Part model, mm, in its own coordinate system. Give positions to 0.01 mm unless a question says otherwise; leave off trailing zeros. Write each loop counter-clockwise with the first axis right and the second up, starting at its lowest first coordinate (ties: lowest second). Pieces come first, ordered by that corner, then holes.
Autodesk Inventor part; units mm, degrees
ref_plane "YZ Plane" through (0, 0, 0) normal (1, 0, 0) x (0, 1, 0)
ref_plane "XZ Plane" through (0, 0, 0) normal (0, 1, 0) x (-1, 0, 0)
ref_plane "XY Plane" through (0, 0, 0) normal (0, 0, 1) x (1, 0, 0)
sketch "Sketch1" plane through (0, 0, 0) normal (0, 1, 0) x (-1, 0, 0)
  line L0 (4.1559, 203.2) -> (4.1559, -203.2)
  line L1 (4.1559, -203.2) -> (156.5559, -291.1882)
  line L2 (4.1559, 203.2) -> (156.5559, 291.1882)
  line L3 (4.1559, 203.2) -> (180.1322, 203.2) construction
  line L4 (156.5559, 291.1882) -> (156.5559, -291.1882)
  point P0 (0, 0)
  point P1 (4.1559, 0)
  dimension "d0" = 120
  dimension "d1" = 30
  dimension "d2" = 406.4
  dimension "d5" = 152.4
extrude "Extrusion1" add sketch "Sketch1" along normal blind 6.35
sketch "Sketch4" plane through (0, 6.35, 0) normal (0, 1, 0) x (1, 0, 0)
  line L0 (-4.1559, -203.2) -> (-4.1559, 203.2)
  point P0 (0, 0)
  point P1 (-80.3559, 0)
  dimension "d12" = 76.2
  dimension "d13" = 203.2
hole "Hole1" at (-80.3559, 6.35, 0) direction (0, -1, 0) diameter 13.4925 end through all
sketch "Sketch5" plane through (0, 6.35, 0) normal (0, 1, 0) x (1, 0, 0)
  line L0 (-1271.2154, -905.4078) -> (-39.3808, -194.2078)
  line L1 (-1258.5154, -927.4048) -> (-1271.2154, -905.4078)
  line L2 (-1258.5154, -927.4048) -> (-26.6808, -216.2048)
  line L3 (-39.3808, -194.2078) -> (-26.6808, -216.2048)
  circle A0 centre (-1049.6741, -711.3284) radius 3.3782
  circle A1 centre (-248.9471, -249.0284) radius 3.3782
  circle A2 centre (-318.2291, -289.0284) radius 3.3782
  circle A3 centre (-1118.9562, -751.3284) radius 3.3782
  line L4 (-127.679, -193.6709) -> (-1227.5312, -828.6709)
  line L5 (-140.379, -171.6739) -> (-127.679, -193.6709)
  line L6 (-140.379, -171.6739) -> (-1240.2312, -806.6739)
  line L7 (-1227.5312, -828.6709) -> (-1240.2312, -806.6739)
  circle A4 centre (-318.2291, 289.0284) radius 3.3782
  circle A5 centre (-1118.9562, 751.3284) radius 3.3782
  circle A6 centre (-1049.6741, 711.3284) radius 3.3782
  circle A7 centre (-248.9471, 249.0284) radius 3.3782
  line L8 (-1227.5312, 828.6709) -> (-127.679, 193.6709)
  line L9 (-1240.2312, 806.6739) -> (-1227.5312, 828.6709)
  line L10 (-1240.2312, 806.6739) -> (-140.379, 171.6739)
  line L11 (-127.679, 193.6709) -> (-140.379, 171.6739)
  line L12 (-39.3808, 194.2078) -> (-1271.2154, 905.4078)
  line L13 (-26.6808, 216.2048) -> (-39.3808, 194.2078)
  line L14 (-26.6808, 216.2048) -> (-1258.5154, 927.4048)
  line L15 (-1271.2154, 905.4078) -> (-1258.5154, 927.4048)
  line L16 (-156.5559, -291.1882) -> (-26.6808, -216.2048)
  line L17 (-39.3808, -194.2078) -> (-156.5559, -261.8588)
  line L18 (-156.5559, 291.1882) -> (-156.5559, -291.1882)
  line L19 (-156.5559, -261.8588) -> (-156.5559, -291.1882)
  line L20 (-156.5559, -210.343) -> (-127.679, -193.6709)
  line L21 (-127.679, -193.6709) -> (-140.379, -171.6739)
  line L22 (-140.379, -171.6739) -> (-156.5559, -181.0136)
  line L23 (-156.5559, -181.0136) -> (-156.5559, -210.343)
  line L24 (-39.3808, -194.2078) -> (-26.6808, -216.2048)
  line L25 (-156.5559, 181.0136) -> (-140.379, 171.6739)
  line L26 (-140.379, 171.6739) -> (-127.679, 193.6709)
  line L27 (-127.679, 193.6709) -> (-156.5559, 210.343)
  line L28 (-156.5559, 210.343) -> (-156.5559, 181.0136)
  line L29 (-156.5559, 261.8588) -> (-39.3808, 194.2078)
  line L30 (-39.3808, 194.2078) -> (-26.6808, 216.2048)
  line L31 (-4.1559, 203.2) -> (-156.5559, 291.1882)
  line L32 (-26.6808, 216.2048) -> (-156.5559, 291.1882)
  line L33 (-156.5559, 291.1882) -> (-156.5559, 261.8588)
  line L34 (-156.5559, 291.1882) -> (-26.6808, 216.2048)
  line L35 (-25.293, -216.5767) -> (-157.5719, -292.9479)
  line L36 (-157.5719, -292.9479) -> (-157.5719, -261.2722)
  line L37 (-157.5719, -261.2722) -> (-39.009, -192.8199)
  line L38 (-39.009, -192.8199) -> (-25.293, -216.5767)
  line L39 (-126.2911, -194.0428) -> (-157.5719, -212.1027)
  line L40 (-157.5719, -212.1027) -> (-157.5719, -180.427)
  line L41 (-157.5719, -180.427) -> (-140.0071, -170.286)
  line L42 (-140.0071, -170.286) -> (-126.2911, -194.0428)
  line L43 (-140.0071, 170.286) -> (-157.5719, 180.427)
  line L44 (-157.5719, 180.427) -> (-157.5719, 212.1027)
  line L45 (-157.5719, 212.1027) -> (-126.2911, 194.0428)
  line L46 (-126.2911, 194.0428) -> (-140.0071, 170.286)
  line L47 (-25.801, 215.6968) -> (-39.009, 192.8199)
  line L48 (-39.009, 192.8199) -> (-157.5719, 261.2722)
  line L49 (-157.5719, 261.2722) -> (-157.5719, 291.1882)
  line L50 (-25.801, 215.6968) -> (-156.5559, 291.1882)
  line L51 (-157.5719, 291.1882) -> (-157.5719, 291.7748)
  line L52 (-157.5719, 291.7748) -> (-156.5559, 291.1882)
  point P0 (0, 0)
  dimension "d22" = 1.016
  dimension "d23" = 1.016
  dimension "d24" = 1.016
  dimension "d25" = 1.016
extrude "Extrusion3" cut sketch "Sketch5" against normal blind 25.4 contours L18 L37 L38 L35 L36 L2 L3 L0 | L18 L2 L36 L0 | L0 L3 L2 L18 | L0 L36 L37 L18 | L36 L2 L1 L0 | L48 L49 L12 L18 | L18 L12 L13 L31 L47 L48 | L43 L44 L10 L18 | L18 L10 L11 L8 L45 L46 L43 | L39 L40 L4 L18 | L18 L4 L5 L6 L41 L42 L39 | L18 L6 L5 L4 | L4 L40 L6 L18 | L4 L7 L6 L40 | L6 L40 L41 L18 | L18 L8 L11 L10 | L10 L44 L8 L18 | L10 L9 L8 L44 | L8 L44 L45 L18 | L18 L14 L13 L12 | L12 L49 L51 L14 L18 | A0 | A1 | A2 | A3 | A4 | A5 | A6 | A7
properties part number "Triangle End"
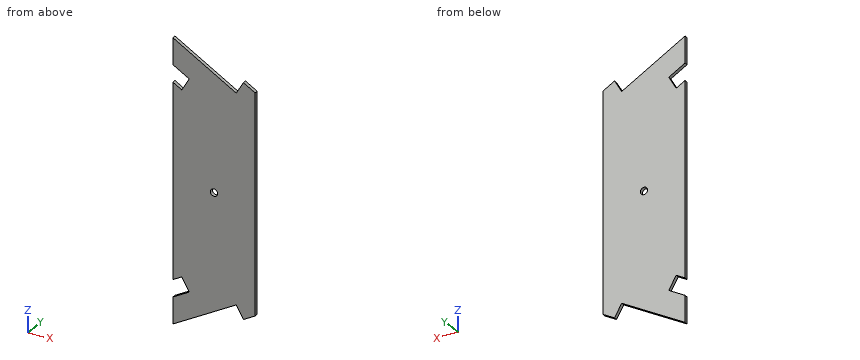
1) Wall check: L1, parallel to X at y = 3, z = 0; L2, parallel to Z at x = -148, y = 4; L3, parallel to Z at x = -86.5, y = 3.75. Give the ranges that are in metal, low to high.
Answers follow:
L1: x = -156.56 to -87.1, -73.61 to -4.16
L2: z = -255.75 to -206.58, -174.9 to 174.9, 206.58 to 255.75
L3: z = -220.24 to -2.79, 2.79 to 220.24
2) Saw through at C-C, the plane x = -63. Write the cut outline in (y, z).
Answers follow:
outline: (0, -206.67) - (6.35, -206.67) - (6.35, 206.67) - (0, 206.67) - close
3) Saw through at A-A, the plane z = 0. Write the cut outline in (x, y), then the cut area to 3 significant figures.
Answers follow:
outline: (-156.56, 0) - (-87.1, 0) - (-87.1, 6.35) - (-156.56, 6.35) - close; (-73.61, 0) - (-4.16, 0) - (-4.16, 6.35) - (-73.61, 6.35) - close
area: 882 mm2
4) Saw through at B-B, the plane y = 2. Write the cut outline in (x, z), then the cut area to 3 significant figures.
Answers follow:
outline: (-156.56, -260.69) - (-39.01, -192.82) - (-25.8, -215.7) - (-4.16, -203.2) - (-4.16, 203.2) - (-25.8, 215.7) - (-39.01, 192.82) - (-156.56, 260.69) - (-156.56, 211.52) - (-126.29, 194.04) - (-140.01, 170.29) - (-156.56, 179.84) - (-156.56, -179.84) - (-140.01, -170.29) - (-126.29, -194.04) - (-156.56, -211.52) - close; hole circle Ø13.49 at (-80.36, 0)
area: 66,100 mm2
5) Pin check, flat tips, straight feed: pin 1 Ø12 at (x, z) = (-80.36, 0) entering from +Y; pin 2 Ø1 at (x, y) = (-28.5, 5) entering from +Z. Stop position of each tip, or through.
Answers follow:
pin 1: passes through
pin 2: stops at z = 211.89
